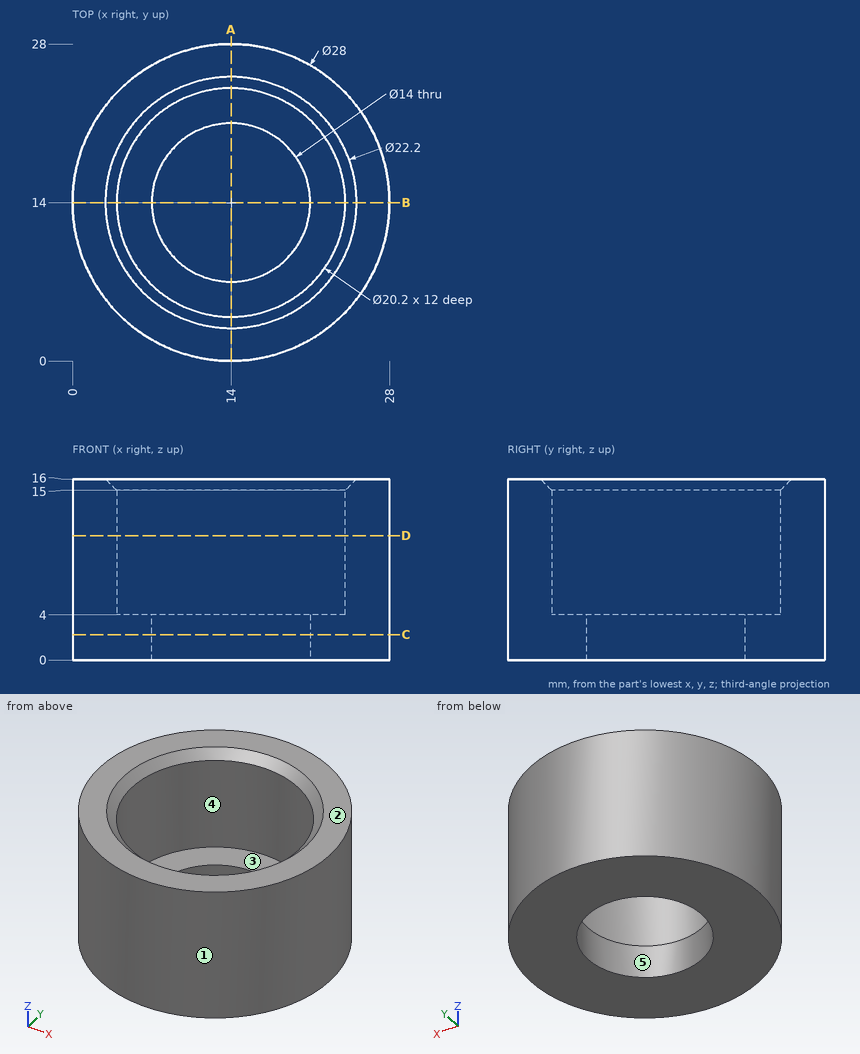
Check sheet for the drawn part. Datum: minimum x, y, z corner. Units: mm. A direction names the side the tool comes from. Coordinates: 2 decimals unless noted, no trailing zeros. Order: outer loops, then holes, each group sorted by start corner. A loop starts at its lowest first (then second) coordinate and runs counter-clockwise, first axis right, second up. Notation, with made-up numbers: M 14.25,-24 L 53.25,-24 A33 ccw 53.25,13 Z; hole C 89.5,85 d2. An arc over 180 degrees is marked long. One line per item, written item: value. Start each with the question number.
Item 1: Mould release check, pull along Y, two halves, no side actions. Record for the marked faces 1, 2 and 3: released by +Y, released by -Y, zero draft, split by the parting line, or undercut.
Item 2: Access from +Z, -Z, +X, -X, +Y, -Y to the whole of each face (thin tool, end or side, straight path). Record for the marked faces 4 and 5.
Item 3: Scan lines: probe 1 along Y at (x, z) = (14, 9.5); probe 2 along Y at (x, z) = (8, 13.25); probe 3 along X at (y, z) = (8.5, 7). Record each from-to range of solid material in increasing order.
Item 4: Sectioned sample at A-A (x = 14). Enter the section's corners in (y, z), then the cut area to 3 significant figures.
Item 5: Sectioned sample at D-D (z = 11). Enter the section's corners in (x, y), then the cut area to 3 significant figures.
Item 6: Sectioned sample at C-C (z = 2.25). Enter the section's corners in (x, y).
Item 7: Gauge pin test, flat ends, axial feed: pin 1 (1.5 mm diameter, centred on x = 20.5, z = 3.5, fed in from -Y); pin 2 (4 mm diameter, centred on x = 8.5, z = 5.5, fed in from -Y); pin 3 (8 mm diameter, centred on y = 7, z = 13.5, fed in from -X); pin 4 (4 mm diameter, centred on x = 12, y = 16.5, fed in from +Z). Record the tip position at first contact, or that the pin passes through.
Conclusion:
1. face 1: split by the parting line
1. face 2: zero draft
1. face 3: undercut
2. face 4: +Z
2. face 5: +Z, -Z
3. probe 1: y = 0 to 3.9, 24.1 to 28
3. probe 2: y = 1.35 to 5.88, 22.12 to 26.65
3. probe 3: x = 1.13 to 5.53, 22.47 to 26.87
4. outline: M 0,0 L 7,0 L 7,4 L 3.9,4 L 3.9,15 L 2.9,16 L 0,16 Z; M 21,0 L 28,0 L 28,16 L 25.1,16 L 24.1,15 L 24.1,4 L 21,4 Z
4. area: 149 mm^2
5. outline: C 14,14 d28; hole C 14,14 d20.2
5. area: 295 mm^2
6. outline: C 14,14 d28; hole C 14,14 d14
7. pin 1: stops at y = 1.24
7. pin 2: stops at y = 0.44
7. pin 3: stops at x = 0.33
7. pin 4: passes through
